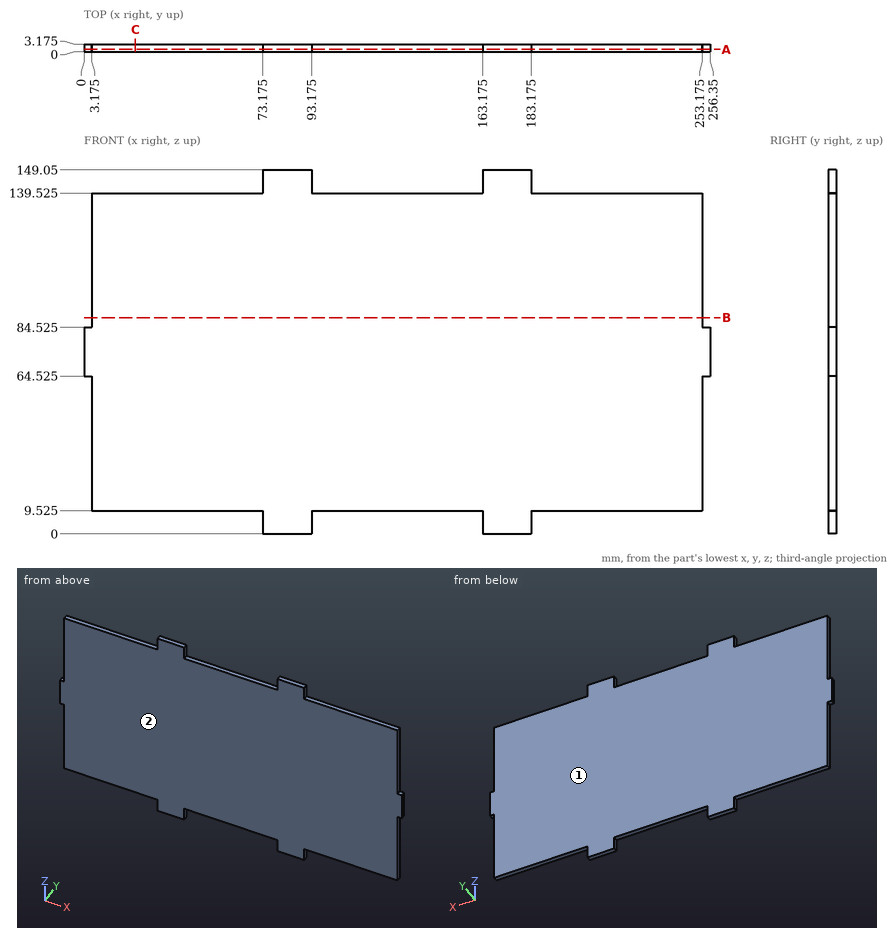
Verification items for this drawing (mm, ordinates from the low corner). Give positions to 0.01 mm unless a question says otherwise; leave off trailing zeros. Loops run counter-clockwise (first coordinate to the right, second up) from the corner with the lowest first, then second, coordinate; pieces in that order, holes last.
1. Cross-section at B-B on z = 88.5. Record the cut outline in (x, y) (3 decimals).
Derived:
outline: (3.175, 0) - (253.175, 0) - (253.175, 3.175) - (3.175, 3.175) - close
2. Release check for a two-part mould opening along Y. For the marked faces 1 and 2 record: +Y half, -Y half, draft (parallel to the pull), parting line (faces both ways), or undercut.
Derived:
face 1: +Y half
face 2: -Y half
3. Cross-section at C-C on x = 21. Record the cut outline in (y, z) (3 decimals).
Derived:
outline: (0, 9.525) - (3.175, 9.525) - (3.175, 139.525) - (0, 139.525) - close
4. Material ranges on probe 1 along X at (y, z) = (0.4, 8.5) (3 decimals); probe 2 along X at (y, z) = (0.4, 59) (3 decimals); probe 3 along Z at (x, y) = (16.5, 0.3) (3 decimals), recorded low to high.
Derived:
probe 1: x = 73.175 to 93.175, 163.175 to 183.175
probe 2: x = 3.175 to 253.175
probe 3: z = 9.525 to 139.525
5. Go/stop test with flat-tipped pins: P1, Ø1, axis at y = 2, z = 34.5, coming from the +X side (3 decimals); P2, Ø1, axis at x = 185.5, y = 1.5, coming from the +Z side (3 decimals); P3, Ø1.6, axis at y = 1.5, z = 146, coming from the -X side (3 decimals). Record where each tip stops, or that it passes through.
Derived:
P1: stops at x = 253.175
P2: stops at z = 139.525
P3: stops at x = 73.175
6. Cross-section at A-A on y = 1. Record the cut outline in (x, z) (3 decimals), and give its area (3 significant figures).
Derived:
outline: (0, 64.525) - (3.175, 64.525) - (3.175, 9.525) - (73.175, 9.525) - (73.175, 0) - (93.175, 0) - (93.175, 9.525) - (163.175, 9.525) - (163.175, 0) - (183.175, 0) - (183.175, 9.525) - (253.175, 9.525) - (253.175, 64.525) - (256.35, 64.525) - (256.35, 84.525) - (253.175, 84.525) - (253.175, 139.525) - (183.175, 139.525) - (183.175, 149.05) - (163.175, 149.05) - (163.175, 139.525) - (93.175, 139.525) - (93.175, 149.05) - (73.175, 149.05) - (73.175, 139.525) - (3.175, 139.525) - (3.175, 84.525) - (0, 84.525) - close
area: 33,400 mm2
